```python
from build123d import *

# Parameters (mm, degrees)
SKETCH_1_W          = 44
SKETCH_1_H          = 25
EXTRUDE_1_DEPTH     = 2
SKETCH_2_W          = 2
SKETCH_2_H          = 25
EXTRUDE_2_DEPTH     = 56
FILLET_1_RADIUS     = 12.5
FILLET_1_LENGTH     = 2
CUT_EXTRUDE_2_REACH = 63.451
SKETCH_3_R          = 4.1
SKETCH_3_R_2        = 1.5
CUT_EXTRUDE_3_REACH = 74.307
SKETCH_4_R          = 4.1
SKETCH_4_R_2        = 1.5
FILLET_2_R          = 2
SKETCH_5_W          = 11
SKETCH_5_H          = 30
CUT_EXTRUDE_4_DEPTH = 62.451200151


with BuildPart() as part:
    # 草图1 → 凸台-拉伸1 (new body)
    with BuildSketch(Plane(origin=(0, 0, 0), x_dir=(1, 0, 0), z_dir=(0, 1, 0))):
        Rectangle(SKETCH_1_W, SKETCH_1_H)
    extrude(amount=-EXTRUDE_1_DEPTH)

    # 草图2 → 凸台-拉伸2 (add)
    with BuildSketch(Plane(origin=(0, 0, 0), x_dir=(1, 0, 0), z_dir=(0, 1, 0))):
        with Locations((-21, 0)):
            Rectangle(SKETCH_2_W, SKETCH_2_H)
    extrude(amount=-EXTRUDE_2_DEPTH)

    # 圆角1: full round fillet: the end face becomes a half cylinder, R = half its width
    fillet_1_face = Plane((22, -1, 0), x_dir=(0, 1, 0), z_dir=(1, 0, 0))  # on the end face: x along it, z out of the body
    fillet_1_slab = fillet_1_face.offset(-FILLET_1_RADIUS / 2) * Box(FILLET_1_LENGTH, 2 * FILLET_1_RADIUS, FILLET_1_RADIUS, mode=Mode.PRIVATE)  # the body's end, R deep
    fillet_1_round = Plane((9.5, -1, 0), x_dir=(1, 0, 0), z_dir=(0, 1, 0)) * Cylinder(FILLET_1_RADIUS, FILLET_1_LENGTH, mode=Mode.PRIVATE)  # its axis R under the face
    add(fillet_1_slab - fillet_1_round, mode=Mode.SUBTRACT)

    # 草图3 → 切除-拉伸2 (cut, up to next)
    with BuildSketch(Plane(origin=(0, 0, 0), x_dir=(1, 0, 0), z_dir=(0, 1, 0)), mode=Mode.PRIVATE) as cut_extrude_2_sk1:
        with Locations(Location((9.5, 0, 0), (0, 0, 270))):
            Circle(SKETCH_3_R)
    cut_extrude_2_tool1 = extrude(cut_extrude_2_sk1.sketch, amount=-CUT_EXTRUDE_2_REACH, mode=Mode.PRIVATE) & part.part
    # 草图3 → 切除-拉伸2 (cut, up to next)
    with BuildSketch(Plane(origin=(0, 0, 0), x_dir=(1, 0, 0), z_dir=(0, 1, 0)), mode=Mode.PRIVATE) as cut_extrude_2_sk2:
        with Locations(Location((2.4, 0, 0), (0, 0, 270))):
            Circle(SKETCH_3_R_2)
    cut_extrude_2_tool2 = extrude(cut_extrude_2_sk2.sketch, amount=-CUT_EXTRUDE_2_REACH, mode=Mode.PRIVATE) & part.part
    # 草图3 → 切除-拉伸2 (cut, up to next)
    with BuildSketch(Plane(origin=(0, 0, 0), x_dir=(1, 0, 0), z_dir=(0, 1, 0)), mode=Mode.PRIVATE) as cut_extrude_2_sk3:
        with Locations(Location((9.5, 7.1, 0), (0, 0, 270))):
            Circle(SKETCH_3_R_2)
    cut_extrude_2_tool3 = extrude(cut_extrude_2_sk3.sketch, amount=-CUT_EXTRUDE_2_REACH, mode=Mode.PRIVATE) & part.part
    # 草图3 → 切除-拉伸2 (cut, up to next)
    with BuildSketch(Plane(origin=(0, 0, 0), x_dir=(1, 0, 0), z_dir=(0, 1, 0)), mode=Mode.PRIVATE) as cut_extrude_2_sk4:
        with Locations(Location((16.6, 0, 0), (0, 0, 270))):
            Circle(SKETCH_3_R_2)
    cut_extrude_2_tool4 = extrude(cut_extrude_2_sk4.sketch, amount=-CUT_EXTRUDE_2_REACH, mode=Mode.PRIVATE) & part.part
    # 草图3 → 切除-拉伸2 (cut, up to next)
    with BuildSketch(Plane(origin=(0, 0, 0), x_dir=(1, 0, 0), z_dir=(0, 1, 0)), mode=Mode.PRIVATE) as cut_extrude_2_sk5:
        with Locations(Location((9.5, -7.1, 0), (0, 0, 270))):
            Circle(SKETCH_3_R_2)
    cut_extrude_2_tool5 = extrude(cut_extrude_2_sk5.sketch, amount=-CUT_EXTRUDE_2_REACH, mode=Mode.PRIVATE) & part.part
    # 草图3 → 切除-拉伸2 (cut, up to next)
    with BuildSketch(Plane(origin=(0, 0, 0), x_dir=(1, 0, 0), z_dir=(0, 1, 0)), mode=Mode.PRIVATE) as cut_extrude_2_sk6:
        with Locations(Location((-9.2, 0, 0), (0, 0, 270))):
            Circle(SKETCH_3_R_2)
    cut_extrude_2_tool6 = extrude(cut_extrude_2_sk6.sketch, amount=-CUT_EXTRUDE_2_REACH, mode=Mode.PRIVATE) & part.part
    add(cut_extrude_2_tool1.solids().sort_by_distance((9.5, 0, 0))[0], mode=Mode.SUBTRACT)
    add(cut_extrude_2_tool2.solids().sort_by_distance((2.4, 0, 0))[0], mode=Mode.SUBTRACT)
    add(cut_extrude_2_tool3.solids().sort_by_distance((9.5, 0, -7.1))[0], mode=Mode.SUBTRACT)
    add(cut_extrude_2_tool4.solids().sort_by_distance((16.6, 0, 0))[0], mode=Mode.SUBTRACT)
    add(cut_extrude_2_tool5.solids().sort_by_distance((9.5, 0, 7.1))[0], mode=Mode.SUBTRACT)
    add(cut_extrude_2_tool6.solids().sort_by_distance((-9.2, 0, 0))[0], mode=Mode.SUBTRACT)

    # 镜向2: part across plane


with BuildPart() as part_1:
    add(part.part)
    add(part.part.mirror(Plane.ZX.offset(-28)))

    # 草图4 → 切除-拉伸3 (cut, up to next)
    with BuildSketch(Plane.ZY.offset(22), mode=Mode.PRIVATE) as cut_extrude_3_sk1:
        with Locations((0, -28)):
            Circle(SKETCH_4_R)
    cut_extrude_3_tool1 = extrude(cut_extrude_3_sk1.sketch, amount=-CUT_EXTRUDE_3_REACH, mode=Mode.PRIVATE) & part_1.part
    # 草图4 → 切除-拉伸3 (cut, up to next)
    with BuildSketch(Plane.ZY.offset(22), mode=Mode.PRIVATE) as cut_extrude_3_sk2:
        with Locations((0, -20.9)):
            Circle(SKETCH_4_R_2)
    cut_extrude_3_tool2 = extrude(cut_extrude_3_sk2.sketch, amount=-CUT_EXTRUDE_3_REACH, mode=Mode.PRIVATE) & part_1.part
    # 草图4 → 切除-拉伸3 (cut, up to next)
    with BuildSketch(Plane.ZY.offset(22), mode=Mode.PRIVATE) as cut_extrude_3_sk3:
        with Locations((7.1, -28)):
            Circle(SKETCH_4_R_2)
    cut_extrude_3_tool3 = extrude(cut_extrude_3_sk3.sketch, amount=-CUT_EXTRUDE_3_REACH, mode=Mode.PRIVATE) & part_1.part
    # 草图4 → 切除-拉伸3 (cut, up to next)
    with BuildSketch(Plane.ZY.offset(22), mode=Mode.PRIVATE) as cut_extrude_3_sk4:
        with Locations((0, -35.1)):
            Circle(SKETCH_4_R_2)
    cut_extrude_3_tool4 = extrude(cut_extrude_3_sk4.sketch, amount=-CUT_EXTRUDE_3_REACH, mode=Mode.PRIVATE) & part_1.part
    # 草图4 → 切除-拉伸3 (cut, up to next)
    with BuildSketch(Plane.ZY.offset(22), mode=Mode.PRIVATE) as cut_extrude_3_sk5:
        with Locations((-7.1, -28)):
            Circle(SKETCH_4_R_2)
    cut_extrude_3_tool5 = extrude(cut_extrude_3_sk5.sketch, amount=-CUT_EXTRUDE_3_REACH, mode=Mode.PRIVATE) & part_1.part
    # 草图4 → 切除-拉伸3 (cut, up to next)
    with BuildSketch(Plane.ZY.offset(22), mode=Mode.PRIVATE) as cut_extrude_3_sk6:
        with Locations((0, -6.9)):
            Circle(SKETCH_4_R_2)
    cut_extrude_3_tool6 = extrude(cut_extrude_3_sk6.sketch, amount=-CUT_EXTRUDE_3_REACH, mode=Mode.PRIVATE) & part_1.part
    # 草图4 → 切除-拉伸3 (cut, up to next)
    with BuildSketch(Plane.ZY.offset(22), mode=Mode.PRIVATE) as cut_extrude_3_sk7:
        with Locations(Location((0, -49.1, 0), (0, 0, 180))):
            Circle(SKETCH_4_R_2)
    cut_extrude_3_tool7 = extrude(cut_extrude_3_sk7.sketch, amount=-CUT_EXTRUDE_3_REACH, mode=Mode.PRIVATE) & part_1.part
    add(cut_extrude_3_tool1.solids().sort_by_distance((-22, -28, 0))[0], mode=Mode.SUBTRACT)
    add(cut_extrude_3_tool2.solids().sort_by_distance((-22, -20.9, 0))[0], mode=Mode.SUBTRACT)
    add(cut_extrude_3_tool3.solids().sort_by_distance((-22, -28, 7.1))[0], mode=Mode.SUBTRACT)
    add(cut_extrude_3_tool4.solids().sort_by_distance((-22, -35.1, 0))[0], mode=Mode.SUBTRACT)
    add(cut_extrude_3_tool5.solids().sort_by_distance((-22, -28, -7.1))[0], mode=Mode.SUBTRACT)
    add(cut_extrude_3_tool6.solids().sort_by_distance((-22, -6.9, 0))[0], mode=Mode.SUBTRACT)
    add(cut_extrude_3_tool7.solids().sort_by_distance((-22, -49.1, 0))[0], mode=Mode.SUBTRACT)

    # 圆角2
    fillet_2_edges = [part_1.edges().sort_by_distance(p)[0] for p in [
        (-22, -56, 0),
        (-22, 0, 0),
    ]]
    fillet(fillet_2_edges, radius=FILLET_2_R)

    # 草图5 → 切除-拉伸4 (cut, through all)
    with BuildSketch(Plane(origin=(0, 0, 0), x_dir=(1, 0, 0), z_dir=(0, 1, 0))):
        with Locations((18.5, 0)):
            Rectangle(SKETCH_5_W, SKETCH_5_H)
    extrude(amount=-CUT_EXTRUDE_4_DEPTH, mode=Mode.SUBTRACT)


solid = part_1.part
```
For this review, take the finished solid that the model builds, in its own axes (mm). A direction names the side the tool comes from. Round coordinates to 2 decimals unless told otherwise and drop trailing zeros. Write each loop counter-clockwise with the first axis right and the second up, starting at its lowest first coordinate (ties: lowest second). Pieces come first, ordered by that corner, then holes. Notation, with made-up numbers: (68.5, 79.5) -> (109.5, 79.5) arc R16 cw to (109.5, 89.5) -> close; hole circle Ø8 at (10.5, 47). An arc over 180 degrees is marked (long way). One line per question, with ' | ' between items. Start each with the question number.
(1) Add section A-A, the plane z = -7.1. Write out the cut boundary in (x, y), plus the area to 3 significant figures.
(2) For line 1 along Y through (x, z) = (0, -7.25); line 2 along Y through (x, z) = (-20.4, 0); line 3 along Y through (x, z) = (-20.5, 0), list the stretches that pass through material, from the lowest coordinate up. Write a range as from..to.
(3) Add section C-C, the plane y = -31.5. Write out the cut boundary in (x, z), plus the area to 3 significant figures.
(4) Tool access review of faces 4 (the face through (13, -1, -7)), 5 (the face through (-4, -54, 0)): name each direction out of +Z, -Z, +X, -X, +Y, -Y from which nothing blocks a thin tool from reaching the whole face with its end or side.
(5) Add section B-B, the plane x = -1. Write out the cut boundary in (y, z).
(6) Add section D-D, the plane x = 6. Write out the cut boundary in (y, z).
(7) Mouldability with a two-part tool opening along X and no side actions: class faces 1 (the face through (-21.43, -0.6, -0.18)), 2 (the face through (-21.014, -5.635, 0.806)), 3 (the face through (0.936, -0.986, -0.325)) as released by +X, released by -X, zero draft, split by the parting line, or undercut.
(8) Insertion check: P1, Ø12, axis at y = -43.5, z = 1.5, coming from the +X side. The pin has a flat end and moves straight along its axis. Give the tip position at first contact, or say it passes through.
Answer list:
1) outline: (-22, -54) arc R2 ccw to (-20, -56) -> (8, -56) -> (8, -54) -> (-20, -54) -> (-20, -29.5) -> (-22, -29.5) -> close; (-22, -26.5) -> (-20, -26.5) -> (-20, -2) -> (8, -2) -> (8, 0) -> (-20, 0) arc R2 ccw to (-22, -2) -> close; (11, -56) -> (13, -56) -> (13, -54) -> (11, -54) -> close; (11, -2) -> (13, -2) -> (13, 0) -> (11, 0) -> close | area: 224 mm²
2) line 1: -56..-54, -2..0 | line 2: -55.96..-50.6, -47.6..-36.6, -33.6..-32.1, -23.9..-22.4, -19.4..-8.4, -5.4..-0.04 | line 3: -55.94..-50.6, -47.6..-36.6, -33.6..-32.1, -23.9..-22.4, -19.4..-8.4, -5.4..-0.06
3) outline: (-22, -12.5) -> (-20, -12.5) -> (-20, -2.14) -> (-22, -2.14) -> close; (-22, 2.14) -> (-20, 2.14) -> (-20, 12.5) -> (-22, 12.5) -> close | area: 41.5 mm²
4) face 4: +Z, -Z, +X, +Y, -Y | face 5: +Z, -Z, +X
5) outline: (-56, -12.5) -> (-54, -12.5) -> (-54, 12.5) -> (-56, 12.5) -> close; (-2, -12.5) -> (0, -12.5) -> (0, 12.5) -> (-2, 12.5) -> close
6) outline: (-56, -12.5) -> (-54, -12.5) -> (-54, -2.14) -> (-56, -2.14) -> close; (-56, 2.14) -> (-54, 2.14) -> (-54, 12.5) -> (-56, 12.5) -> close; (-2, -12.5) -> (0, -12.5) -> (0, -2.14) -> (-2, -2.14) -> close; (-2, 2.14) -> (0, 2.14) -> (0, 12.5) -> (-2, 12.5) -> close
7) face 1: released by -X | face 2: zero draft | face 3: undercut
8) P1: x = -20
